from build123d import *

# Parameters (mm, degrees)
BOSS_EXTRUDE1_DEPTH = 4
BOSS_EXTRUDE2_START = 12
SKETCH3_R           = 3.5
BOSS_EXTRUDE2_DEPTH = 12
SKETCH4_W           = 16
SKETCH4_H           = 3
BOSS_EXTRUDE3_DEPTH = 15
FILLET3_R           = 10
FILLET5_R           = 14


with BuildPart() as part:
    # Sketch2 → Boss-Extrude1 (new body)
    with BuildSketch(Plane.XY):
        with BuildLine():
            Line((-2, 41.178043508), (2, 41.178043508))
            Line((2, 41.178043508), (2, 27.712303128))
            ThreePointArc((2, 27.712303128), (2.036985125, 26.659599059), (2.147758114, 25.612086241))
            Line((2.147758114, 25.612086241), (3.94525946, 12.900577758))
            ThreePointArc((3.94525946, 12.900577758), (3.94789108, 12.8818827), (3.950499168, 12.863184344))
            Line((3.950499168, 12.863184344), (5.5790973, 1.133209829))
            Line((5.5790973, 1.133209829), (5.736432971, 0))
            Line((5.736432971, 0), (5.5790973, -1.133209829))
            Line((5.5790973, -1.133209829), (3.860857289, -13.50882979))
            ThreePointArc((3.860857289, -13.50882979), (2.625757677, -15.790400529), (0.196011829, -16.7))
            Line((0.196011829, -16.7), (-0.196011829, -16.7))
            ThreePointArc((-0.196011829, -16.7), (-2.625757677, -15.790400529), (-3.860857289, -13.50882979))
            Line((-3.860857289, -13.50882979), (-5.5790973, -1.133209829))
            Line((-5.5790973, -1.133209829), (-5.736432971, 0))
            Line((-5.736432971, 0), (-5.5790973, 1.133209829))
            Line((-5.5790973, 1.133209829), (-3.950499168, 12.863184344))
            ThreePointArc((-3.950499168, 12.863184344), (-3.94789108, 12.8818827), (-3.94525946, 12.900577758))
            Line((-3.94525946, 12.900577758), (-2.147758114, 25.612086241))
            ThreePointArc((-2.147758114, 25.612086241), (-2.036985125, 26.659599059), (-2, 27.712303128))
            Line((-2, 27.712303128), (-2, 41.178043508))
        make_face()
        with BuildLine():
            Line((-3.598099755, -0.858166699), (-1.879859743, -13.23378666))
            ThreePointArc((-1.879859743, -13.23378666), (-1.312381543, -14.282075919), (-0.196011829, -14.7))
            Line((-0.196011829, -14.7), (0.196011829, -14.7))
            ThreePointArc((0.196011829, -14.7), (1.312381543, -14.282075919), (1.879859743, -13.23378666))
            Line((1.879859743, -13.23378666), (3.598099755, -0.858166699))
            Line((3.598099755, -0.858166699), (3.717248239, 0))
            Line((3.717248239, 0), (3.598099755, 0.858166699))
            Line((3.598099755, 0.858166699), (1.879859743, 13.23378666))
            ThreePointArc((1.879859743, 13.23378666), (1.312381543, 14.282075919), (0.196011829, 14.7))
            Line((0.196011829, 14.7), (-0.196011829, 14.7))
            ThreePointArc((-0.196011829, 14.7), (-1.312381543, 14.282075919), (-1.879859743, 13.23378666))
            Line((-1.879859743, 13.23378666), (-3.598099755, 0.858166699))
            Line((-3.598099755, 0.858166699), (-3.717248239, 0))
            Line((-3.717248239, 0), (-3.598099755, -0.858166699))
        make_face(mode=Mode.SUBTRACT)
    extrude(amount=-BOSS_EXTRUDE1_DEPTH)

    # Sketch3 → Boss-Extrude2 (add)
    with BuildSketch(Plane.XY.offset(BOSS_EXTRUDE2_START)):
        with BuildLine():
            Line((-3.950499168, 12.863184344), (-5.736432971, 0))
            Line((-5.736432971, 0), (-3.860857289, -13.50882979))
            ThreePointArc((-3.860857289, -13.50882979), (-2.625757677, -15.790400529), (-0.196011829, -16.7))
            Line((-0.196011829, -16.7), (0.196011829, -16.7))
            ThreePointArc((0.196011829, -16.7), (2.625757677, -15.790400529), (3.860857289, -13.50882979))
            Line((3.860857289, -13.50882979), (5.736432971, 0))
            Line((5.736432971, 0), (3.950499168, 12.863184344))
            ThreePointArc((3.950499168, 12.863184344), (3.94789108, 12.8818827), (3.94525946, 12.900577758))
            Line((3.94525946, 12.900577758), (2.147758114, 25.612086241))
            ThreePointArc((2.147758114, 25.612086241), (2.036985125, 26.659599059), (2, 27.712303128))
            Line((2, 27.712303128), (2, 41.178043508))
            Line((2, 41.178043508), (-2, 41.178043508))
            Line((-2, 41.178043508), (-2, 27.712303128))
            ThreePointArc((-2, 27.712303128), (-2.036985125, 26.659599059), (-2.147758114, 25.612086241))
            Line((-2.147758114, 25.612086241), (-3.94525946, 12.900577758))
            ThreePointArc((-3.94525946, 12.900577758), (-3.94789108, 12.8818827), (-3.950499168, 12.863184344))
        make_face()
        Circle(SKETCH3_R, mode=Mode.SUBTRACT)
    extrude(amount=-BOSS_EXTRUDE2_DEPTH)

    # Sketch4 → Boss-Extrude3 (add)
    with BuildSketch(Plane.ZY.offset(2)):
        with Locations((4, 39.678043508)):
            Rectangle(SKETCH4_W, SKETCH4_H)
    extrude(amount=BOSS_EXTRUDE3_DEPTH)

    # Fillet3
    fillet3_edges = [part.edges().sort_by_distance(p)[0] for p in [
        (-2, 38.178043508, 4),
    ]]
    fillet(fillet3_edges, radius=FILLET3_R)

    # Fillet5
    fillet5_edges = [part.edges().sort_by_distance(p)[0] for p in [
        (2, 41.178043508, 4),
    ]]
    fillet(fillet5_edges, radius=FILLET5_R)


solid = part.part
Part model, mm, in its own coordinate system. A direction names the side the tool comes from. Coordinates: 2 decimals unless noted, no trailing zeros. Order: outer loops, then holes, each group sorted by start corner. A loop starts at its lowest first (then second) coordinate and runs counter-clockwise, first axis right, second up. Notation, with made-up numbers: M 35,10.5 L 92,10.5 A30 ccw 92,40.5 Z; hole C 11.25,58.25 d2. An arc over 180 degrees is marked long. One line per question, with ' | ' between items.
Q1. 3-axis set-ups, long thin cutter, end or side, ignore diameter. For faces 1 (the face through (1.299, -14.293, -1.972)), 2 (the face through (-2.036, 26.674, 4.112)), 3 (the face through (3.233, -1.341, 6.084)): which of +Z, -Z, +X, -X, +Y, -Y reach the whole face in a straight line?
A:
face 1: -Z | face 2: +Z, -Z, -X | face 3: +Z, -Z
Q2. Drill centre lines: line 1 (Y direction, x = 0, z = 9.75); line 2 (Z direction, x = 1, y = -10); line 3 (X direction, y = 1, z = 0.25). Where is each one in solid material? Low to high.
A:
line 1: y = -16.7 to -3.5, 3.5 to 34.4 | line 2: z = 0 to 12 | line 3: x = -5.6 to -3.35, 3.35 to 5.6
Q3. Pin check, flat tips, straight feed: P1, Ø2.5, axis at x = -15, z = 6.5, coming from the -Y side; P2, Ø1, axis at x = -7, z = -0.5, coming from the -Y side; P3, Ø6, axis at y = 24.5, z = 6.5, coming from the +X side. Stop position of each tip, or through.
A:
P1: stops at y = 38.18 | P2: stops at y = 36.53 | P3: stops at x = 2.73
Q4. Slice it at D-D (y = 20). Give the cut face in (x, z), and give its area (3 significant figures).
A:
outline: M -2.94,-4 L 2.94,-4 L 2.94,12 L -2.94,12 Z | area: 94.1 mm^2
Q5. Two-plate mould, pull along X, no slides. Class faces 4 (the face through (1.6, 3.5, 0)), 5 (the face through (-14, 38.178, 4)), 6 (the face through (2.05, 26.51, 4.11)): +X half, -X half, draft (parallel to the pull), parting line (faces both ways), or undercut.
A:
face 4: undercut | face 5: draft | face 6: +X half
Q6. Slice it at C-C (y = -9.5). Give the cut face in (x, z), and give its area (3 significant figures).
A:
outline: M -4.42,-4 L -2.4,-4 L -2.4,0 L 2.4,0 L 2.4,-4 L 4.42,-4 L 4.42,12 L -4.42,12 Z | area: 122 mm^2
Q7. Slice it at B-B (x = 4.5). Give the cut face in (y, z), and give its area (3 significant figures).
A:
outline: M -8.91,-4 L 8.91,-4 L 8.91,12 L -8.91,12 Z | area: 285 mm^2
Q8. Slice it at A-A (y = 6.5). Give the cut face in (x, z).
A:
outline: M -4.83,-4 L -2.81,-4 L -2.81,0 L 2.81,0 L 2.81,-4 L 4.83,-4 L 4.83,12 L -4.83,12 Z
